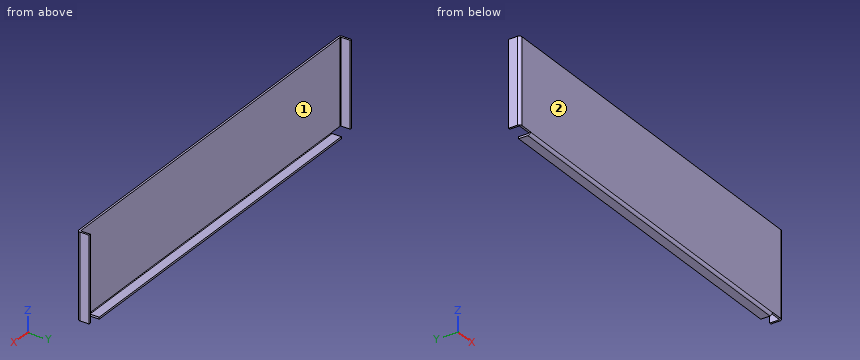
from build123d import *

# Parameters (mm, degrees)
SKETCH1_W               = 614.68
SKETCH1_H               = 138.6205
BASE_FLANGE1_DEPTH      = 3.175
EDGE_FLANGE1_DEPTH      = 138.6205
EDGE_FLANGE1_BEND_DEPTH = 138.6205
EDGE_FLANGE2_DEPTH      = 578.136


# Sheet-metal steps are written as plain solids
with BuildPart() as part:
    # Sketch1 → Base-Flange1 (new body)
    with BuildSketch(Plane(origin=(0, 0, 0), x_dir=(1, 0, 0), z_dir=(0, 1, 0))):
        Rectangle(SKETCH1_W, SKETCH1_H)
    extrude(amount=-BASE_FLANGE1_DEPTH)

    # Edge-Flange1 section (across the edge) → Edge-Flange1 (add)
    with BuildSketch(Plane(origin=(-310.388, 0, -69.31025), x_dir=(1, 0, 0), z_dir=(0, 0, 1))):
        with BuildLine():
            Line((-3.175, 1), (-3.175, 15.875))
            Line((-3.175, 15.875), (0, 15.875))
            Line((0, 15.875), (0, 1))
            ThreePointArc((0, 1), (0.292893219, 0.292893219), (1, 0))
            Line((1, 0), (3.048, 0))
            Line((3.048, 0), (3.048, -3.175))
            Line((3.048, -3.175), (1, -3.175))
            ThreePointArc((1, -3.175), (-1.952170811, -1.952170811), (-3.175, 1))
        make_face()
    extrude(amount=EDGE_FLANGE1_DEPTH)

    # Edge-Flange1 section 2 (across the edge) → Edge-Flange1 bend (add)
    with BuildSketch(Plane(origin=(310.388, 0, 69.31025), x_dir=(-1, 0, 0), z_dir=(0, 0, -1))):
        with BuildLine():
            Line((-3.175, 1), (-3.175, 15.875))
            Line((-3.175, 15.875), (0, 15.875))
            Line((0, 15.875), (0, 1))
            ThreePointArc((0, 1), (0.292893219, 0.292893219), (1, 0))
            Line((1, 0), (3.048, 0))
            Line((3.048, 0), (3.048, -3.175))
            Line((3.048, -3.175), (1, -3.175))
            ThreePointArc((1, -3.175), (-1.952170811, -1.952170811), (-3.175, 1))
        make_face()
    extrude(amount=EDGE_FLANGE1_BEND_DEPTH)

    # Edge-Flange2 section (across the edge) → Edge-Flange2 (add)
    with BuildSketch(Plane(origin=(289.068, 0, -70.58025), x_dir=(0, 0, 1), z_dir=(-1, 0, 0))):
        with BuildLine():
            Line((-3.175, 1), (-3.175, 15.875))
            Line((-3.175, 15.875), (0, 15.875))
            Line((0, 15.875), (0, 1))
            ThreePointArc((0, 1), (0.292893219, 0.292893219), (1, 0))
            Line((1, 0), (1.27, 0))
            Line((1.27, 0), (1.27, -3.175))
            Line((1.27, -3.175), (1, -3.175))
            ThreePointArc((1, -3.175), (-1.952170811, -1.952170811), (-3.175, 1))
        make_face()
    extrude(amount=EDGE_FLANGE2_DEPTH)


solid = part.part
Work out the finished part from the listing and answer in its coordinate system (mm). Face numbers are marked on the shaded views. Give positions to 0.01 mm unless a question says otherwise; leave off trailing zeros. Loops run counter-clockwise (first coordinate to the right, second up) from the corner with the lowest first, then second, coordinate; pieces in that order, holes last. Notation, with made-up numbers: (70, 61) - (129, 61) arc R8 ccw to (129, 68) - close; hole circle Ø11 at (67.5, -6). An arc over 180 degrees is marked (long way). Answer in a Markdown table with one row per item.
(1) Section C-C (z = -13) is taken. Give the vertices of the cut face in (x, y) (3 decimals).
Results list:
| item | result |
|---|---|
| outline | (-313.563, 1) arc R4.175 ccw to (-309.388, -3.175) - (309.388, -3.175) arc R4.175 ccw to (313.563, 1) - (313.563, 15.875) - (310.388, 15.875) - (310.388, 1) arc R1 cw to (309.388, 0) - (-309.388, 0) arc R1 cw to (-310.388, 1) - (-310.388, 15.875) - (-313.563, 15.875) - close |
(2) Consider L1, parallel to X at y = 7.75, z = -13; L2, parallel to Y at x = 206, z = -44 (3 decimals); L3, parallel to Z at x = 24.5, y = 14. Determine where each line is inside the solid, lowest interval first. Write a range as [from, to].
Results list:
| item | result |
|---|---|
| L1 | x = [-313.56, -310.39], [310.39, 313.56] |
| L2 | y = [-3.175, 0] |
| L3 | z = [-73.76, -70.58] |
(3) A flat-ended cylindrical pin translates along its axis: pin 1 Ø1.3 at (y, z) = (8.5, -71.5) entering from -X. Find the tip coordinate at first contact, or state that the pin passes through.
Results list:
| item | result |
|---|---|
| pin 1 | stops at x = -289.07 |
(4) For a pull along X with two mould halves and no side action, classify the marked faces 1 and 2 as pulls with the +X half, pulls with the -X half, needs draft (parallel to the pull), parting line crosses it, or undercut.
Results list:
| item | result |
|---|---|
| face 1 | undercut |
| face 2 | needs draft |
(5) Section B-B (x = 94.5) is taken. Give the vertices of the cut face in (y, z) (3 decimals).
Results list:
| item | result |
|---|---|
| outline | (-3.175, -69.58) arc R4.175 ccw to (1, -73.755) - (15.875, -73.755) - (15.875, -70.58) - (1, -70.58) arc R1 cw to (0, -69.58) - (0, 69.31) - (-3.175, 69.31) - close |
(6) Section A-A (y = 6.5) is taken. Give the vertices of the cut face in (x, z).
Results list:
| item | result |
|---|---|
| outline | (-313.56, -69.31) - (-310.39, -69.31) - (-310.39, 69.31) - (-313.56, 69.31) - close; (-289.07, -73.76) - (289.07, -73.76) - (289.07, -70.58) - (-289.07, -70.58) - close; (310.39, -69.31) - (313.56, -69.31) - (313.56, 69.31) - (310.39, 69.31) - close |
